Autodesk Inventor part; units mm, degrees
ref_plane "YZ Plane" through (0, 0, 0) normal (1, 0, 0) x (0, 1, 0)
ref_plane "XZ Plane" through (0, 0, 0) normal (0, 1, 0) x (-1, 0, 0)
ref_plane "XY Plane" through (0, 0, 0) normal (0, 0, 1) x (1, 0, 0)
sketch "Sketch1" plane through (0, 0, 0) normal (0, 0, 1) x (1, 0, 0)
  arc A0 (-5.9989, 1.3197) -> (6.0793, 1.2962) centre (0.0364, -0.6546) ccw
  arc A1 (2.3687, 12.7903) -> (-2.2437, 12.7993) centre (0.0611, 12.0454) ccw
  line L0 (-2.2437, 12.7993) -> (-5.9989, 1.3197)
  line L1 (2.3687, 12.7903) -> (6.0793, 1.2962)
  dimension "d0" = 12.7
  dimension "d8" = 12.7
extrude "Extrusion1" add sketch "Sketch1" along normal blind 6.35
sketch "Sketch2" plane through (0, 0, 6.35) normal (0, 0, 1) x (1, 0, 0)
  arc A0 (-5.2619, 3.4373) -> (5.5303, 3.1215) centre (0.0364, -0.6546) ccw
  circle A1 centre (0.0364, -0.6546) radius 1.5875
  dimension "d4" = 3.175
extrude "Extrusion2" add sketch "Sketch2" along normal blind 25.4
properties part number "cam"
Model file for the job. Use its own axes, mm. A direction names the side the tool comes from. Coordinates: 2 decimals unless noted, no trailing zeros. Loops run counter-clockwise (first coordinate to the right, second up) from the corner with the lowest first, then second, coordinate; pieces in that order, holes last. Notation, with made-up numbers: (83.5, 23) - (140.5, 23) arc R18 cw to (140.5, 33) - close; hole circle Ø8 at (3, -10.5). An arc over 180 degrees is marked (long way). Answer as a JSON object with one key per item and string values. Group by question number.
(1) Cut at D-D (x = -3.5). Give the cut face in (y, z).
(2) Probe line 1 along Z through (x, y) = (-1.5, 4); line 2 along X through (y, z) = (3.75, 3); line 3 along X through (y, z) = (-0.75, 18). List the from-to ranges inside material, lowest first.
(3) Cut at B-B (y = -0.25). Give the cut face in (x, z), then the cut area to 3 significant figures.
(4) Cut at A-A (x = 1). Give the cut face in (y, z), then the cut area to 3 significant figures.
(5) Cut at C-C (z = 7). Give the cut face in (x, y) (1 decimal), then the cut area to 3 significant figures.
(6) Flat gauge pins, fed straight in: pin 1 (4 mm diameter, centred on x = -2, y = 7.5, fed in from +Z); pin 2 (2 mm diameter, centred on x = -2, z = 15.5, fed in from -Y); pin 3 (2 mm diameter, centred on x = 3, z = 5.5, fed in from +Y); pin 4 (6 mm diameter, centred on x = 5, z = 16.5, fed in from +Y). Where does each tip first touch, or does it go through?
(7) Tool access for faces 1 (the face through (1.55, -1.13, 18.87)), 2 (the face through (0, -1, 31.75)): list every direction of +Z, -Z, +X, -X, +Y, -Y with a clear straight run to the whole face (end or side of a thin tool).
Geometry says:
{
 "1": {"outline": "(-5.93, 0) - (8.96, 0) - (8.96, 6.35) - (-5.93, 6.35) - close"},
 "2": {"line 1": "z = 0 to 6.35", "line 2": "x = -5.2 to 5.29", "line 3": "x = -1.55 to 1.62"},
 "3": {"outline": "(-6.3, 0) - (6.37, 0) - (6.37, 6.35) - (1.57, 6.35) - (1.57, 31.75) - (-1.5, 31.75) - (-1.5, 6.35) - (-6.3, 6.35) - close", "area": "158 mm^2"},
 "4": {"outline": "(-6.93, 0) - (14.28, 0) - (14.28, 6.35) - (0.61, 6.35) - (0.61, 31.75) - (-1.92, 31.75) - (-1.92, 6.35) - (-6.93, 6.35) - close", "area": "199 mm^2"},
 "5": {"outline": "circle Ø3.2 at (0, -0.7)", "area": "7.92 mm^2"},
 "6": {"pin 1": "stops at z = 6.35", "pin 2": "stops at y = -1.86", "pin 3": "stops at y = 13.5", "pin 4": "passes through"},
 "7": {"face 1": "+Z", "face 2": "+Z, +X, -X, +Y, -Y"}
}
